Build history of the part. All positions in model axes, mm. Face numbers are marked on the shaded views. A direction names the side the tool comes from. Round coordinates to 2 decimals unless told otherwise and drop trailing zeros. Write each loop counter-clockwise with the first axis right and the second up, starting at its lowest first coordinate (ties: lowest second). Pieces come first, ordered by that corner, then holes.
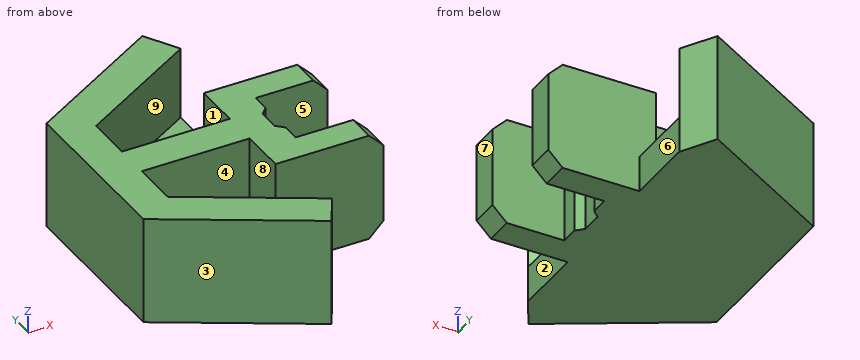
from build123d import *

# Parameters (mm, degrees)
F1_DEPTH  = 38.1
F2_SIZE   = 5.08
F4_DEPTH  = 38.1
F6_DEPTH  = 12.7
F7_W      = 38.1
F7_H      = 16.5227
F7_H_2    = 16.557139
F8_DEPTH  = 25.4
F10_DEPTH = 38.101


with BuildPart() as f1:
    # F0 (on Top) → F1 (new body)
    with BuildSketch(Plane.XY):
        Polygon((0, 0), (0, 25.4254), (25.4, 25.4254), (25.4, 35.5854), (-50.8, 35.5854), (-50.8, -10.16), (25.4, -10.16), (25.4, 0), align=None)
    extrude(amount=F1_DEPTH)

    # F2
    f2_edges = [f1.edges().sort_by_distance(p)[0] for p in [
        (25.4, -5.08, 0),
        (25.4, 30.5054, 0),
        (25.4, -5.08, 38.1),
        (25.4, 30.5054, 38.1),
    ]]
    chamfer(f2_edges, length=F2_SIZE)

    # F3 (on face) → F4 (join)
    with BuildSketch(Plane(origin=(0, 0, 0), x_dir=(1, 0, 0), z_dir=(0, 0, -1))):
        Polygon((-50.8, -35.5854), (-50.8, 10.16), (-6.805909, 35.56), (-13.155909, 46.558523), (-63.5, 17.492348), (-63.5, 10.16), (-63.5, -35.5854), (-63.5, -44.245531), (-13.730856, -72.97976), (-6.805909, -60.9854), align=None)
    extrude(amount=-F4_DEPTH)

    # F5 (on face) → F6 (join)
    with BuildSketch(Plane(origin=(0, 0, 0), x_dir=(1, 0, 0), z_dir=(0, 0, -1))):
        Polygon((-6.805909, -60.9854), (-6.805909, 35.56), (-50.8, 10.16), (-50.8, -35.5854), align=None)
    extrude(amount=-F6_DEPTH)

    # F7 (on face) → F8 (cut, through all)
    with BuildSketch(Plane.XY.offset(38.1)):
        with Locations((-31.75, -1.89865)):
            Rectangle(F7_W, F7_H)
        with Locations((-31.75, 27.306831)):
            Rectangle(F7_W, F7_H_2)
    extrude(amount=-F8_DEPTH, mode=Mode.SUBTRACT)

    # F9 (on face) → F10 (cut, through all)
    with BuildSketch(Plane.XY.offset(38.1)):
        Polygon((-2.54, 16.5227), (-2.54, 8.9027), (0, 6.3627), (0, 19.0627), align=None)
    extrude(amount=-F10_DEPTH, mode=Mode.SUBTRACT)


solid = f1.part
1) Pin check, flat tips, straight feed: pin 1 Ø14 at (y, z) = (50.5, 8) entering from +X; pin 2 Ø5 at (y, z) = (4.5, 27.5) entering from +X; pin 3 Ø1 at (x, z) = (-51.5, 33) entering from +Y. Stop position of each tip, or through.
Results:
pin 1: stops at x = -6.81
pin 2: stops at x = 0
pin 3: stops at y = 51.46
2) Slice it at A-A (x = 10.5). Write the cut outline in (y, z).
Results:
outline: (-10.16, 0) - (0, 0) - (0, 38.1) - (-10.16, 38.1) - close; (25.43, 0) - (35.59, 0) - (35.59, 38.1) - (25.43, 38.1) - close
3) Slice it at D-D (x = -18). Write the cut outline in (y, z), plus the area to 3 significant figures.
Results:
outline: (-43.76, 0) - (70.51, 0) - (70.51, 38.1) - (54.52, 38.1) - (54.52, 12.7) - (19.03, 12.7) - (19.03, 38.1) - (6.36, 38.1) - (6.36, 12.7) - (-29.1, 12.7) - (-29.1, 38.1) - (-43.76, 38.1) - close
area: 2,550 mm2
4) Slice it at B-B (z = 3). Write the cut outline in (x, y), plus the area to 3 significant figures.
Results:
outline: (-63.5, -17.49) - (-13.16, -46.56) - (-6.81, -35.56) - (-6.81, -10.16) - (23.32, -10.16) - (23.32, 0) - (0, 0) - (0, 6.36) - (-2.54, 8.9) - (-2.54, 16.52) - (0, 19.06) - (0, 25.43) - (23.32, 25.43) - (23.32, 35.59) - (-6.81, 35.59) - (-6.81, 60.99) - (-13.73, 72.98) - (-63.5, 44.25) - close
area: 6,010 mm2
5) Mould opens along X. For the marked faces 1, 2, 3 and 4 say: released by +X, released by -X, zero draft, split by the parting line, or undercut.
Results:
face 1: undercut
face 2: released by +X
face 3: released by -X
face 4: undercut
6) Which spindle directions (+Z, -Z, +X, -X, +Y, -Y) get a long thin tool onto all of the face, cutting with end or side? Do the marked faces 5, 6, 7, 8 and 9. Say none if no direction does.
Results:
face 5: +Z, -Z, +X
face 6: +Z, -Z, +X, +Y
face 7: +Z, -Z, +X, +Y, -Y
face 8: +Z
face 9: +Z, +X
7) Slice it at C-C (y = -8). Write the cut outline in (x, z).
Results:
outline: (-63.5, 0) - (20.32, 0) - (25.4, 5.08) - (25.4, 33.02) - (20.32, 38.1) - (-12.7, 38.1) - (-12.7, 12.7) - (-50.8, 12.7) - (-50.8, 38.1) - (-63.5, 38.1) - close
8) Wall check: L1, parallel to Y at x = 17, z = 4; L2, parallel to X at y = 32.5, z = 19.5; L3, parallel to Y at x = -31, z = 24. Give the ranges that are in metal, low to high.
Results:
L1: y = -10.16 to 0, 25.43 to 35.59
L2: x = -63.5 to -50.8, -12.7 to 25.4
L3: y = -36.26 to -21.59, 6.36 to 19.03, 47.02 to 63.01
